Verification items for the finished model (mm, model axes). A direction names the side the tool comes from. Round coordinates to 2 decimals unless told otherwise and drop trailing zeros. Write each loop counter-clockwise with the first axis right and the second up, starting at its lowest first coordinate (ties: lowest second). Pieces come first, ordered by that corner, then holes. Notation, with made-up numbers: (65.5, 38.25) - (99.5, 38.25) arc R36 cw to (99.5, 73.25) - close; hole circle Ø11 at (-17.5, -27.75). An arc over 180 degrees is marked (long way). Answer as a JSON object with one key per item and string values.
```python
from build123d import *

# Parameters (mm, degrees)
ESQUISSE1_R             = 1.435
ESQUISSE1_R_2           = 1.5
BOSS_EXTRU_2_DEPTH      = 2.5
BOSS_EXTRU_3_DEPTH      = 6.5
ESQUISSE3_R             = 4
ENL_V_MAT_EXTRU_1_DEPTH = 10


with BuildPart() as part:
    # Esquisse1 → Boss.-Extru.2 (new body)
    with BuildSketch(Plane.XY):
        with BuildLine():
            Line((22.427498376, 0), (24.908638492, -9.449680852))
            ThreePointArc((24.908638492, -9.449680852), (28.04, -11.865), (31.171361508, -9.449680852))
            Line((31.171361508, -9.449680852), (33.652501624, 0))
            ThreePointArc((33.652501624, 0), (43.38, 14.385), (33.652501624, 28.77))
            Line((33.652501624, 28.77), (31.171361508, 38.219680852))
            ThreePointArc((31.171361508, 38.219680852), (28.04, 40.635), (24.908638492, 38.219680852))
            Line((24.908638492, 38.219680852), (22.427498376, 28.77))
            Line((22.427498376, 28.77), (4.087498376, 28.77))
            Line((4.087498376, 28.77), (0, 23.555))
            Line((0, 23.555), (0, 5.215))
            Line((0, 5.215), (4.087498376, 0))
            Line((4.087498376, 0), (22.427498376, 0))
        make_face()
        with Locations((28.04, 37.3975)):
            Circle(ESQUISSE1_R, mode=Mode.SUBTRACT)
        with Locations((28.04, -8.6275)):
            Circle(ESQUISSE1_R, mode=Mode.SUBTRACT)
        with Locations((28.04, 30.6)):
            Circle(ESQUISSE1_R_2, mode=Mode.SUBTRACT)
        with Locations((28.04, -1.83)):
            Circle(ESQUISSE1_R_2, mode=Mode.SUBTRACT)
    extrude(amount=BOSS_EXTRU_2_DEPTH)

    # Esquisse2 → Boss.-Extru.3 (add)
    with BuildSketch(Plane.XY.offset(2.5)):
        with BuildLine():
            Line((4.087498376, 28.77), (33.652501624, 28.77))
            ThreePointArc((33.652501624, 28.77), (43.38, 14.385), (33.652501624, 0))
            Line((33.652501624, 0), (4.087498376, 0))
            Line((4.087498376, 0), (0, 5.215))
            Line((0, 5.215), (0, 23.555))
            Line((0, 23.555), (4.087498376, 28.77))
        make_face()
    extrude(amount=BOSS_EXTRU_3_DEPTH)

    # Esquisse3 → Enlèv. mat.-Extru.1 (cut)
    with BuildSketch(Plane.XY.offset(9)):
        with Locations((28.04, 14.385)):
            Circle(ESQUISSE3_R)
    extrude(amount=-ENL_V_MAT_EXTRU_1_DEPTH, mode=Mode.SUBTRACT)


solid = part.part
```
Q1. Material ranges on line 1 along Y through (x, z) = (29, 1); line 2 along X through (y, z) = (15, 6); line 3 along Z through (x, y) = (27.5, 35), recorded low to high. Write a range as [from, to].
Geometry check:
{"line 1": "y = [-11.72, -9.69], [-7.56, -2.98], [-0.68, 10.5], [18.27, 29.45], [31.75, 36.33], [38.46, 40.49]", "line 2": "x = [0, 24.09], [31.99, 43.37]", "line 3": "z = [0, 2.5]"}
Q2. Release check for a two-part mould opening along Y. For faces 1 (the flat face through (32.43, 33.43, 1.23)), 2 (the flat face through (22, 15, 9)), 3 (the cylindrical face through (26.54, 30.67, 1.23)) record: released by +Y, released by -Y, zero draft, split by the parting line, or undercut.
Geometry check:
{"face 1": "released by +Y", "face 2": "zero draft", "face 3": "undercut"}
Q3. Section check B-B, the plane z = 5.5. Record the cut outline in (x, y) (1 decimal), then the cut area to 3 significant figures.
Geometry check:
{"outline": "(0, 5.2) - (4.1, 0) - (33.7, 0) arc R15.5 ccw to (33.7, 28.8) - (4.1, 28.8) - (0, 23.6) - close; hole circle Ø8 at (28, 14.4)", "area": "1,100 mm2"}
Q4. Section check C-C, the plane y = -2.5. Record the cut outline in (x, z), then the cut area to 3 significant figures.
Geometry check:
{"outline": "(23.08, 0) - (26.7, 0) - (26.7, 2.5) - (23.08, 2.5) - close; (29.38, 0) - (33, 0) - (33, 2.5) - (29.38, 2.5) - close", "area": "18.1 mm2"}
Q5. Set-up check for faces 4 (the flat face through (28, -5, 2.5)), 5 (the flat face through (19, 28.77, 4)), 6 (the flat face through (19, 0, 4)), 7 (the flat face through (32.395, -4.791, 1.232)): record each of +Z, -Z, +X, -X, +Y, -Y from which the full face is reachable in a straight line by a thin tool's end or side.
Geometry check:
{"face 4": "+Z, +X, -X, -Y", "face 5": "+Z, -X, +Y", "face 6": "+Z, -X, -Y", "face 7": "+Z, -Z, +X, -Y"}
Q6. Gauge pin test, flat ends, axial feed: P1, Ø3.5, axis at x = 28, y = -8, coming from the +Z side; P2, Ø2.5, axis at x = 28.04, y = -1.83, coming from the +Z side; P3, Ø4, axis at x = 33, z = 6.5, coming from the +Y side; P4, Ø4, axis at y = 33, z = 1, coming from the +X side. Record the tip position at first contact, or that the pin passes through.
Geometry check:
{"P1": "stops at z = 2.5", "P2": "passes through", "P3": "stops at y = 28.77", "P4": "stops at x = 33.07"}
Q7. Section check D-D, the plane z = 1.5. Record the cut outline in (x, y) (1 decimal), then the cut area to 3 significant figures.
Geometry check:
{"outline": "(0, 5.2) - (4.1, 0) - (22.4, 0) - (24.9, -9.4) arc R3.2 ccw to (31.2, -9.4) - (33.7, 0) arc R15.5 ccw to (33.7, 28.8) - (31.2, 38.2) arc R3.2 ccw to (24.9, 38.2) - (22.4, 28.8) - (4.1, 28.8) - (0, 23.6) - close; hole circle Ø8 at (28, 14.4); hole circle Ø3 at (28, -1.8); hole circle Ø3 at (28, 30.6); hole circle Ø2.9 at (28, -8.6); hole circle Ø2.9 at (28, 37.4)", "area": "1,260 mm2"}
Q8. Section check A-A, the plane x = 28.04. State how many separate pieces and enclosed holes the cut face has, then the cut area to 3 significant figures.
Geometry check:
{"separate pieces": "6", "enclosed holes": "0", "area": "217 mm2"}
